from build123d import *

# Parameters (mm, degrees)
SKETCH2_W                                           = 150
SKETCH2_H                                           = 40
BOSS_EXTRUDE1_DEPTH                                 = 20
SKETCH3_R                                           = 13.5
CUT_EXTRUDE1_DEPTH                                  = 13
LPATTERN1_COUNT                                     = 5
LPATTERN1_PITCH                                     = 30
CBORE_FOR_M4_HEX_SOCKET_HEAD_CAP_SCREW1_D           = 4.5
CBORE_FOR_M4_HEX_SOCKET_HEAD_CAP_SCREW1_CBORE_D     = 8
CBORE_FOR_M4_HEX_SOCKET_HEAD_CAP_SCREW1_CBORE_DEPTH = 4.4
LPATTERN2_COUNT                                     = 2
LPATTERN2_PITCH                                     = 120
SKETCH7_W                                           = 181.12901383
SKETCH7_H                                           = 4
CUT_EXTRUDE3_DEPTH                                  = 13


with BuildPart() as part:
    # Sketch2 → Boss-Extrude1 (new body)
    with BuildSketch(Plane(origin=(0, 0, 0), x_dir=(1, 0, 0), z_dir=(0, 1, 0))):
        Rectangle(SKETCH2_W, SKETCH2_H)
    extrude(amount=BOSS_EXTRUDE1_DEPTH)

    # Sketch3 → Cut-Extrude1 (cut)
    with BuildSketch(Plane(origin=(0, 20, 0), x_dir=(1, 0, 0), z_dir=(0, 1, 0))):
        with Locations(Location((-60, 0, 0), (0, 0, 270))):
            Circle(SKETCH3_R)
    cut_extrude1 = extrude(amount=-CUT_EXTRUDE1_DEPTH, mode=Mode.SUBTRACT)

    # LPattern1: Cut-Extrude1 ×5
    with Locations(*[(i * LPATTERN1_PITCH, 0, 0) for i in range(1, LPATTERN1_COUNT)]):
        add(cut_extrude1, mode=Mode.SUBTRACT)

    # CBORE for M4 Hex Socket Head Cap Screw1 (through all)
    with Locations(Plane(origin=(0, 7, 0), x_dir=(-1, 0, 0), z_dir=(0, 1, 0))):
        with Locations((60, 0)):
            cbore_for_m4_hex_socket_head_cap_screw1 = CounterBoreHole(CBORE_FOR_M4_HEX_SOCKET_HEAD_CAP_SCREW1_D / 2, CBORE_FOR_M4_HEX_SOCKET_HEAD_CAP_SCREW1_CBORE_D / 2, CBORE_FOR_M4_HEX_SOCKET_HEAD_CAP_SCREW1_CBORE_DEPTH)

    # LPattern2: CBORE for M4 Hex Socket Head Cap Screw1 ×2
    with Locations(*[(i * LPATTERN2_PITCH, 0, 0) for i in range(1, LPATTERN2_COUNT)]):
        add(cbore_for_m4_hex_socket_head_cap_screw1, mode=Mode.SUBTRACT)

    # Sketch7 → Cut-Extrude3 (cut)
    with BuildSketch(Plane(origin=(0, 20, 0), x_dir=(1, 0, 0), z_dir=(0, 1, 0))):
        Rectangle(SKETCH7_W, SKETCH7_H)
    extrude(amount=-CUT_EXTRUDE3_DEPTH, mode=Mode.SUBTRACT)


solid = part.part
Design review of the part built by this model. Coordinates are the model's own, in mm. A direction names the side the tool comes from. Coordinates: 2 decimals unless noted, no trailing zeros. Write each loop counter-clockwise with the first axis right and the second up, starting at its lowest first coordinate (ties: lowest second). Pieces come first, ordered by that corner, then holes. Notation, with made-up numbers: (9, 53) - (30, 53) arc R19 cw to (30, 57) - close; hole circle Ø7 at (31, 81.5). An arc over 180 degrees is marked (long way). One line per item, written item: value.
1) Mouldability with a two-part tool opening along Z and no side actions: class faces 4 (the face through (56.185, 4.831, 1.201)), 5 (the face through (-1, 10, 20)), 6 (the face through (-1, 0, 0)) as +Z half, -Z half, draft (parallel to the pull), parting line (faces both ways), or undercut.
Answer sheet:
face 4: undercut
face 5: +Z half
face 6: draft
2) To check wall thickness, follow probe 1 along Z at (x, y) = (60, 1.5); probe 2 along X at (y, z) = (4, 1); probe 3 along X at (y, z) = (11.5, -9.5). State the ranges of each line that lie inside material, in increasing order.
Answer sheet:
probe 1: z = -20 to -2.25, 2.25 to 20
probe 2: x = -75 to -63.87, -56.13 to 56.13, 63.87 to 75
probe 3: x = -75 to -69.59, -50.41 to -39.59, -20.41 to -9.59, 9.59 to 20.41, 39.59 to 50.41, 69.59 to 75
3) For faces 1 (the face through (-45, 14, -2)), 2 (the face through (-75, 5, 0)), 3 (the face through (-59.731, 13.591, -13.497)), list the 3-axis set-ups (+Z, -Z, +X, -X, +Y, -Y) from which the entire face can be reached by the end or side of a thin tool; tool diameter is ignored.
Answer sheet:
face 1: +X, -X, +Y
face 2: +Z, -Z, -X, +Y, -Y
face 3: +Y
4) Add section B-B (y = 13.25). State the section outline as (x, z) points, plus the area to 3 significant figures.
Answer sheet:
outline: (-75, -20) - (75, -20) - (75, -2) - (73.35, -2) arc R13.5 cw to (46.65, -2) - (43.35, -2) arc R13.5 cw to (16.65, -2) - (13.35, -2) arc R13.5 cw to (-13.35, -2) - (-16.65, -2) arc R13.5 cw to (-43.35, -2) - (-46.65, -2) arc R13.5 cw to (-73.35, -2) - (-75, -2) - close; (-75, 2) - (-73.35, 2) arc R13.5 cw to (-46.65, 2) - (-43.35, 2) arc R13.5 cw to (-16.65, 2) - (-13.35, 2) arc R13.5 cw to (13.35, 2) - (16.65, 2) arc R13.5 cw to (43.35, 2) - (46.65, 2) arc R13.5 cw to (73.35, 2) - (75, 2) - (75, 20) - (-75, 20) - close
area: 3,080 mm2
5) Add section A-A (z = 0). State the section outline as (x, y) points, plus the area to 3 significant figures.
Answer sheet:
outline: (-75, 0) - (-62.25, 0) - (-62.25, 2.6) - (-64, 2.6) - (-64, 7) - (-75, 7) - close; (-57.75, 0) - (57.75, 0) - (57.75, 2.6) - (56, 2.6) - (56, 7) - (-56, 7) - (-56, 2.6) - (-57.75, 2.6) - close; (62.25, 0) - (75, 0) - (75, 7) - (64, 7) - (64, 2.6) - (62.25, 2.6) - close
area: 956 mm2
6) Add section C-C (x = 60). State the section outline as (y, z) points, plus the area to 3 significant figures.
Answer sheet:
outline: (0, -20) - (20, -20) - (20, -13.5) - (7, -13.5) - (7, -4) - (2.6, -4) - (2.6, -2.25) - (0, -2.25) - close; (0, 2.25) - (2.6, 2.25) - (2.6, 4) - (7, 4) - (7, 13.5) - (20, 13.5) - (20, 20) - (0, 20) - close
area: 402 mm2
7) Add section D-D (x = 45). State the section outline as (y, z) points.
Answer sheet:
outline: (0, -20) - (20, -20) - (20, -2) - (7, -2) - (7, 2) - (20, 2) - (20, 20) - (0, 20) - close
8) Insertion check: pin 1 (12 mm diameter, centred on x = -8.5, z = 12, fed in from -Y); pin 2 (1 mm diameter, centred on x = -0.5, z = 7.5, fed in from +Y). Each pin has a flat end and moves straight along its axis. Give the tip position at first contact, or say it passes through.
Answer sheet:
pin 1: stops at y = 0
pin 2: stops at y = 7
